Build history of the part. All positions in model axes, mm. Face numbers are marked on the shaded views. A direction names the side the tool comes from. Round coordinates to 2 decimals unless told otherwise and drop trailing zeros. Write each loop counter-clockwise with the first axis right and the second up, starting at its lowest first coordinate (ties: lowest second). Pieces come first, ordered by that corner, then holes.
1) Saw through at D-D (x = 20). Write the cut outline in (y, z).
2) Saw through at A-A (x = 65). Write the cut outline in (y, z), plus the area to 3 significant figures.
3) Pull direction Z, two halves, no side cores. Call the marked faces 4, 5 and 6: +Z half, -Z half, draft (parallel to the pull), parting line (faces both ways), or undercut.
4) Which spindle directions (+Z, -Z, +X, -X, +Y, -Y) get a long thin tool onto all of the face, cutting with end or side? Do the marked faces 1, 2 and 3. Say none if no direction does.
5) Flat gauge pins, fed straight in: pin 1 (1.2 mm diameter, centred on x = 93, z = 115.5, fed in from +Y); pin 2 (0.6 mm diameter, centred on y = 56, z = 42, fed in from +X); pin 3 (1.2 mm diameter, centred on x = 92.5, z = 58.5, fed in from +Y). Where does each tip first touch, or does it go through?
6) Saw through at B-B (y = 20). Write the cut outline in (x, z), plus the area to 3 significant figures.
7) Saw through at C-C (z = 47). Write the cut outline in (x, y).
8) Wall check: probe 1 along Z at (x, y) = (56.5, 46); probe 2 along Y at (x, z) = (35.5, 83); probe 3 along Z at (x, y) = (69.5, 52). Give the ranges that are in metal, low to high.
from build123d import *

# Parameters (mm, degrees)
F1_DEPTH    = 118
F4_DEPTH    = 61
F5_SIZE     = 2.49999
F6_R        = 5
F7_SIZE     = 3
F8_R        = 2.5
F9_T1_DEPTH = 118


# Not quite as in the source:
# - a fillet or chamfer that OpenCascade refuses, or shapes differently, is made with other operations: its cross-section is extruded or revolved along the edge and cut away or added
# - a fillet or chamfer is up to 0.001 mm smaller than in the source, because OpenCascade refuses the exact size


with BuildPart() as f1:
    # F0 (on Top) → F1 (new body)
    with BuildSketch(Plane.XY):
        Polygon((15.3875516164, 8.1571814393), (15.3875516164, 4.6571814393), (93.7208858402, 4.6571814393), (93.7208858402, 42.6571814393), (89.2208858402, 42.6571814393), (89.2208858402, 55.4571814393), (90.7208858402, 55.4571814393), (90.7208858402, 58.6571814393), (22.7208858402, 58.6571814393), (22.7208858402, 8.1571814393), align=None)
    extrude(amount=F1_DEPTH)

    # F3 (on face) → F4 (cut)
    with BuildSketch(Plane.YZ.offset(93.7208858402)):
        with BuildLine():
            Line((51.1571814393, 113), (42.6571814393, 113))
            Line((42.6571814393, 113), (42.6571814393, 61.5))
            Line((42.6571814393, 61.5), (51.1571814393, 61.5))
            ThreePointArc((51.1571814393, 61.5), (52.9249483923, 62.232233047), (53.6571814393, 64))
            Line((53.6571814393, 64), (53.6571814393, 110.5))
            ThreePointArc((53.6571814393, 110.5), (52.9249483923, 112.267766953), (51.1571814393, 113))
        make_face()
        with BuildLine():
            Line((42.6571814393, 61.5), (42.6571814393, 113))
            Line((42.6571814393, 113), (12.1571814393, 113))
            ThreePointArc((12.1571814393, 113), (10.3894144863, 112.267766953), (9.6571814393, 110.5))
            Line((9.6571814393, 110.5), (9.6571814393, 64))
            ThreePointArc((9.6571814393, 64), (10.3894144863, 62.232233047), (12.1571814393, 61.5))
            Line((12.1571814393, 61.5), (42.6571814393, 61.5))
        make_face()
        with BuildLine():
            Line((12.1571814393, 5), (42.6571814393, 5))
            Line((42.6571814393, 5), (42.6571814393, 56.5))
            Line((42.6571814393, 56.5), (12.1571814393, 56.5))
            ThreePointArc((12.1571814393, 56.5), (10.3894144863, 55.767766953), (9.6571814393, 54))
            Line((9.6571814393, 54), (9.6571814393, 7.5))
            ThreePointArc((9.6571814393, 7.5), (10.3894144863, 5.732233047), (12.1571814393, 5))
        make_face()
        with BuildLine():
            Line((42.6571814393, 56.5), (42.6571814393, 5))
            Line((42.6571814393, 5), (51.1571814393, 5))
            ThreePointArc((51.1571814393, 5), (52.9249483923, 5.732233047), (53.6571814393, 7.5))
            Line((53.6571814393, 7.5), (53.6571814393, 54))
            ThreePointArc((53.6571814393, 54), (52.9249483923, 55.767766953), (51.1571814393, 56.5))
            Line((51.1571814393, 56.5), (42.6571814393, 56.5))
        make_face()
    extrude(amount=-F4_DEPTH, mode=Mode.SUBTRACT)

    # F5 (size 2.5 in the source; OpenCascade refuses exactly that, so slightly less here)
    f5_edges = [f1.edges().sort_by_distance(p)[0] for p in [
        (32.720886, 52.924948, 112.267767),
        (32.720886, 31.657181, 113),
        (32.720886, 10.389414, 112.267767),
        (32.720886, 9.657181, 87.25),
        (32.720886, 10.389414, 62.232233),
        (32.720886, 31.657181, 61.5),
        (32.720886, 52.924948, 62.232233),
        (32.720886, 53.657181, 87.25),
        (32.720886, 10.389414, 5.732233),
        (32.720886, 31.657181, 5),
        (32.720886, 52.924948, 5.732233),
        (32.720886, 53.657181, 30.75),
        (32.720886, 52.924948, 55.767767),
        (32.720886, 31.657181, 56.5),
        (32.720886, 10.389414, 55.767767),
        (32.720886, 9.657181, 30.75),
    ]]
    chamfer(f5_edges, length=F5_SIZE)

    # F6
    f6_edges = [f1.edges().sort_by_distance(p)[0] for p in [
        (56.720886, 58.657181, 118),
        (56.720886, 58.657181, 0),
    ]]
    fillet(f6_edges, radius=F6_R)

    # F7
    f7_edges = [f1.edges().sort_by_distance(p)[0] for p in [
        (89.220886, 42.657181, 59),
        (89.220886, 42.657181, 2.5),
        (89.220886, 42.657181, 115.5),
    ]]
    chamfer(f7_edges, length=F7_SIZE)

    # F8
    f8_edges = [f1.edges().sort_by_distance(p)[0] for p in [
        (93.720886, 4.657181, 59),
    ]]
    fillet(f8_edges, radius=F8_R)

    # F9: fillet of radius 2 on 1 edges, made by hand

    # F9_s2 → F9_t1 (cut)
    with BuildSketch(Plane.XY):
        with BuildLine():
            ThreePointArc((90.7208858402, 56.6571814393), (90.1350994026, 58.0713950017), (88.7208858402, 58.6571814393))
            Line((88.7208858402, 58.6571814393), (90.7208858402, 58.6571814393))
            Line((90.7208858402, 58.6571814393), (90.7208858402, 56.6571814393))
        make_face()
    extrude(amount=F9_T1_DEPTH, mode=Mode.SUBTRACT)


solid = f1.part
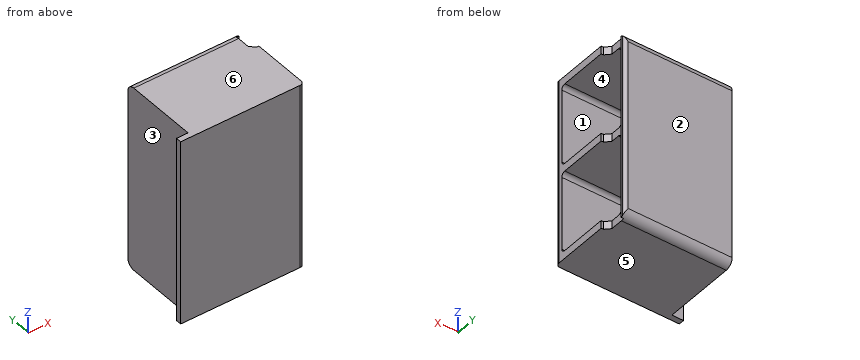
Evaluation:
1. outline: (4.66, 0) - (8.16, 0) - (8.16, 118) - (4.66, 118) - close
2. outline: (4.66, 0) - (53.66, 0) arc R5 ccw to (58.66, 5) - (58.66, 113) arc R5 ccw to (53.66, 118) - (4.66, 118) - close; hole (9.66, 7.5) arc R2.5 ccw to (12.16, 5) - (51.16, 5) arc R2.5 ccw to (53.66, 7.5) - (53.66, 54) arc R2.5 ccw to (51.16, 56.5) - (12.16, 56.5) arc R2.5 ccw to (9.66, 54) - close; hole (9.66, 64) arc R2.5 ccw to (12.16, 61.5) - (51.16, 61.5) arc R2.5 ccw to (53.66, 64) - (53.66, 110.5) arc R2.5 ccw to (51.16, 113) - (12.16, 113) arc R2.5 ccw to (9.66, 110.5) - close
2. area: 1,840 mm2
3. face 4: undercut
3. face 5: -Z half
3. face 6: +Z half
4. face 1: +X
4. face 2: +Z, -Z, +X, -X, +Y
4. face 3: +Z, -Z, -X, +Y
5. pin 1: stops at y = 42.66
5. pin 2: stops at x = 90.72
5. pin 3: stops at y = 42.98
6. outline: (22.72, 0) - (93.72, 0) - (93.72, 5) - (35.22, 5) - (32.72, 7.5) - (32.72, 54) - (35.22, 56.5) - (93.72, 56.5) - (93.72, 61.5) - (35.22, 61.5) - (32.72, 64) - (32.72, 110.5) - (35.22, 113) - (93.72, 113) - (93.72, 118) - (22.72, 118) - close
6. area: 2,110 mm2
7. outline: (15.39, 4.66) - (91.22, 4.66) arc R2.5 ccw to (93.72, 7.16) - (93.72, 9.66) - (35.22, 9.66) - (32.72, 12.16) - (32.72, 51.16) - (35.22, 53.66) - (89.22, 53.66) - (89.22, 55.46) - (90.72, 55.46) - (90.72, 56.66) arc R2 ccw to (88.72, 58.66) - (22.72, 58.66) - (22.72, 8.16) - (15.39, 8.16) - close
8. probe 1: z = 0 to 5, 56.5 to 61.5, 113 to 118
8. probe 2: y = 4.66 to 9.66, 53.66 to 58.66
8. probe 3: z = 0 to 5.15, 56.35 to 61.65, 112.85 to 118
